from build123d import *

# Parameters (mm, degrees)
F0_W      = 158
F0_H      = 115
F1_DEPTH  = 20
F2_T      = -2
F3_W      = 2
F3_H      = 2
F3_H_2    = 111
F4_DEPTH  = 20
F5_W      = 2
F5_H      = 1
F6_DEPTH  = 18
F7_W      = 10
F7_H      = 2
F8_DEPTH  = 2
F21_W     = 21
F21_H     = 2
F22_DEPTH = 1


with BuildPart() as f1:
    # F0 (on Top) → F1 (new body)
    with BuildSketch(Plane.XY):
        with Locations((-40.1476950792, 0.7924512029)):
            Rectangle(F0_W, F0_H)
    extrude(amount=F1_DEPTH)

    # F2
    f2_openings = [f1.faces().sort_by_distance(p)[0] for p in [
        (-40.147695, 0.792451, 20),
    ]]
    offset(amount=F2_T, openings=f2_openings)

    # F3 (on face) → F4 (join)
    with BuildSketch(Plane.XY.offset(20)):
        with Locations((-66.1476950792, 57.2924512029)):
            Rectangle(F3_W, F3_H)
        with Locations((-66.1476950792, -55.7075487971)):
            Rectangle(F3_W, F3_H)
        with Locations((-14.1476950792, 57.2924512029)):
            Rectangle(F3_W, F3_H)
        with Locations((-14.1476950792, -55.7075487971)):
            Rectangle(F3_W, F3_H)
        with Locations((-14.1476950792, 0.7924512029)):
            Rectangle(F3_W, F3_H_2)
        with Locations((-66.1476950792, 0.7924512029)):
            Rectangle(F3_W, F3_H_2)
    extrude(amount=-F4_DEPTH)

    # F5 (on face) → F6 (cut)
    with BuildSketch(Plane.XY.offset(20)):
        with Locations((37.8523049208, 55.7924512029)):
            Rectangle(F5_W, F5_H)
        with Locations((37.8523049208, -54.2075487971)):
            Rectangle(F5_W, F5_H)
    extrude(amount=-F6_DEPTH, mode=Mode.SUBTRACT)

    # F7 (on face) → F8 (cut)
    with BuildSketch(Plane.XY.offset(20)):
        with Locations((-92.1476950792, 57.2924512029)):
            Rectangle(F7_W, F7_H)
        with Locations((11.8523049208, 57.2924512029)):
            Rectangle(F7_W, F7_H)
        with Locations((-40.1753512025, 57.2924512029)):
            Rectangle(F7_W, F7_H)
    extrude(amount=-F8_DEPTH, mode=Mode.SUBTRACT)

    # F9 (on face) → F10 (revolve)
    with BuildSketch(Plane.YZ.offset(-97.1476950792)):
        with BuildLine():
            ThreePointArc((56.9494204277, 18.3330443139), (57.6831089294, 18.3597761792), (58.0424512029, 19))
            ThreePointArc((58.0424512029, 19), (57.9330206868, 19.3900906769), (57.6366625729, 19.6663471563))
            Line((57.6366625729, 19.6663471563), (56.9494204277, 18.3330443139))
        make_face()
    revolve(axis=Axis((-97.1476950792, 57.2930415003, 18.9996957351), (0, -0.4581616098, -0.8888689101)))

    # F11 (on face) → F12 (revolve)
    with BuildSketch(Plane(origin=(-87.1476950792, 0, 0), x_dir=(0, -1, 0), z_dir=(-1, 0, 0))):
        with BuildLine():
            ThreePointArc((-56.5737668636, 18.7855406321), (-56.5503214115, 18.8916331565), (-56.5424512029, 19))
            ThreePointArc((-56.5424512029, 19), (-57.1849084822, 19.7422496637), (-58.0116100381, 19.2128627954))
            Line((-58.0116100381, 19.2128627954), (-56.5737668636, 18.7855406321))
        make_face()
    revolve(axis=Axis((-87.1476950792, 57.2926884509, 18.9992017138), (0, -0.9585627073, -0.2848816178)))

    # F13 (on face) → F14 (revolve)
    with BuildSketch(Plane(origin=(-35.1753512025, 0, 0), x_dir=(0, -1, 0), z_dir=(-1, 0, 0))):
        with BuildLine():
            ThreePointArc((-56.5544690905, 18.8662749021), (-56.5454617169, 18.9328679819), (-56.5424512029, 19))
            ThreePointArc((-56.5424512029, 19), (-57.2299686819, 19.7473927579), (-58.0320403617, 19.1245306231))
            Line((-58.0320403617, 19.1245306231), (-56.5544690905, 18.8662749021))
        make_face()
    revolve(axis=Axis((-35.1753512025, 57.2932547261, 18.9954027626), (0, -0.9850665855, -0.172173814)))

    # F15 (on face) → F16 (revolve)
    with BuildSketch(Plane.YZ.offset(-45.1753512025)):
        with BuildLine():
            ThreePointArc((56.9089305888, 18.3554754166), (57.6631664167, 18.3480258976), (58.0424512029, 19))
            ThreePointArc((58.0424512029, 19), (57.9443668734, 19.3708179586), (57.675768647, 19.6446454351))
            Line((57.675768647, 19.6446454351), (56.9089305888, 18.3554754166))
        make_face()
    revolve(axis=Axis((-45.1753512025, 57.2923496179, 19.0000604259), (0, -0.5112253785, -0.8594466897)))

    # F17 (on face) → F18 (revolve)
    with BuildSketch(Plane.YZ.offset(6.8523049208)):
        with BuildLine():
            ThreePointArc((56.8813847049, 18.3726848206), (57.648962161, 18.3401515805), (58.0424512029, 19))
            ThreePointArc((58.0424512029, 19), (57.9515038931, 19.35797982), (57.7007190655, 19.6291401691))
            Line((57.7007190655, 19.6291401691), (56.8813847049, 18.3726848206))
        make_face()
    revolve(axis=Axis((6.8523049208, 57.2910518852, 19.0009124949), (0, -0.546224262, -0.8376389769)))

    # F19 (on face) → F20 (revolve)
    with BuildSketch(Plane(origin=(16.8523049208, 0, 0), x_dir=(0, -1, 0), z_dir=(-1, 0, 0))):
        with BuildLine():
            ThreePointArc((-56.7624630169, 18.4693282345), (-56.5996340771, 18.7127641557), (-56.5424512029, 19))
            ThreePointArc((-56.5424512029, 19), (-57.0069017432, 19.6935138831), (-57.8250152191, 19.5280867056))
            Line((-57.8250152191, 19.5280867056), (-56.7624630169, 18.4693282345))
        make_face()
    revolve(axis=Axis((16.8523049208, 57.293739118, 18.99870747), (0, -0.7083702312, -0.7058410696)))

    # F21 (on face) → F22 (cut)
    with BuildSketch(Plane.XZ.offset(56.7075487971)):
        with Locations((-40.1476950792, 9.5)):
            Rectangle(F21_W, F21_H)
    extrude(amount=-F22_DEPTH, mode=Mode.SUBTRACT)


solid = f1.part
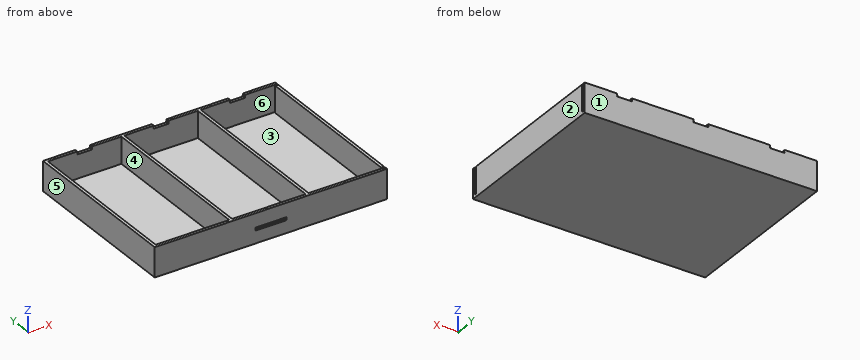
Design review of the part built by this model. Coordinates are the model's own, in mm. Face numbers are marked on the shaded views. A direction names the side the tool comes from. Give positions to 0.01 mm unless a question says otherwise; leave off trailing zeros. Loops run counter-clockwise (first coordinate to the right, second up) from the corner with the lowest first, then second, coordinate; pieces in that order, holes last. Notation, with made-up numbers: M 51,38 L 79,38 A18 ccw 79,47 Z; hole C 11,85 d8. An arc over 180 degrees is marked long. Write item = value, one per line.
Q1. We need section A-A (z = 12.5). Give the boundary of the cut face in (x, y), plus the area to 3 significant figures.
Output values:
outline = M -119.15,-56.71 L 38.85,-56.71 L 38.85,-54.71 L -13.15,-54.71 L -13.15,56.29 L 38.85,56.29 L 38.85,58.29 L -119.15,58.29 Z; M 36.85,-53.71 L 38.85,-53.71 L 38.85,55.29 L 36.85,55.29 Z; hole M -117.15,-54.71 L -67.15,-54.71 L -67.15,56.29 L -117.15,56.29 Z; hole M -65.15,-54.71 L -15.15,-54.71 L -15.15,56.29 L -65.15,56.29 Z
area = 1,520 mm^2
Q2. Insertion check: pin 1 (3 mm diameter, centred on x = 9.5, y = 37, fed in from +Z); pin 2 (1.5 mm diameter, centred on x = -36, z = 9.5, fed in from -Y). Each pin has a flat end and moves straight along its axis. Give the tip position at first contact, or say it passes through.
Output values:
pin_1 = 2
pin_2 = -55.71
Q3. Draft analysis for pull direction X (two halves, no side actions). For the marked faces 1, 2 and 3, state which applies: +X half, -X half, draft (parallel to the pull), parting line (faces both ways), or undercut.
Output values:
face_1 = draft
face_2 = +X half
face_3 = undercut
Q4. For the marked faces 4, 5 and 6, list the 3-axis set-ups (+Z, -Z, +X, -X, +Y, -Y) from which the entire face can be reached by the end or side of a thin tool; tool diameter is ignored.
Output values:
face_4 = +Z
face_5 = +Z, -Z, -X, +Y, -Y
face_6 = +Z, +X
Q5. We need section C-C (y = 17). Give the boundary of the cut face in (x, z).
Output values:
outline = M -119.15,0 L 38.85,0 L 38.85,20 L 36.85,20 L 36.85,2 L -13.15,2 L -13.15,20 L -15.15,20 L -15.15,2 L -65.15,2 L -65.15,20 L -67.15,20 L -67.15,2 L -117.15,2 L -117.15,20 L -119.15,20 Z
Q6. We need section D-D (x = -32). Give the boundary of the cut face in (y, z).
Output values:
outline = M -56.71,0 L 58.29,0 L 58.29,20 L 56.29,20 L 56.29,2 L -54.71,2 L -54.71,20 L -56.71,20 L -56.71,10.5 L -55.71,10.5 L -55.71,8.5 L -56.71,8.5 Z
Q7. To check wall thickness, follow line 1 (X direction, y = 23, z = 15); line 2 (Y direction, x = -16, z = 3.5); line 3 (Z direction, x = -59, y = -37). State the ranges of each line that lie inside material, in increasing order. Write a range as [from, to].
Output values:
line_1 = [-119.15, -117.15], [-67.15, -65.15], [-15.15, -13.15], [36.85, 38.85]
line_2 = [-56.71, -54.71], [56.29, 58.29]
line_3 = [0, 2]
Q8. We need section B-B (x = -90). Give the boundary of the cut face in (y, z).
Output values:
outline = M -56.71,0 L 58.29,0 L 58.29,18 L 56.29,18 L 56.29,2 L -54.71,2 L -54.71,20 L -56.71,20 Z
